Part model, mm, in its own coordinate system. A direction names the side the tool comes from. Round coordinates to 2 decimals unless told otherwise and drop trailing zeros. Write each loop counter-clockwise with the first axis right and the second up, starting at its lowest first coordinate (ties: lowest second). Pieces come first, ordered by that corner, then holes. Notation, with made-up numbers: (86.5, -10) -> (103.5, -10) arc R30 ccw to (103.5, 13) -> close; hole circle Ø5 at (-34.75, 12.5). An arc over 180 degrees is marked (long way). Use CSV: the item, a comma, the result in double quotes. Start each with the question number.
```python
from build123d import *

# Parameters (mm, degrees)
F0_W      = 114.3
F0_H      = 127
F1_DEPTH  = 304.8
F2_SIZE2  = 22.86
F2_SIZE   = 22.86
F4_D      = 63.5
F5_R      = 44.45
F5_R_2    = 31.75
F6_DEPTH  = 63.5
F8_W      = 55.88
F8_H      = 99.06
F9_DEPTH  = 147.32
F11_DEPTH = 55.88
F13_DEPTH = 302.261
F14_R     = 22.86
F15_DEPTH = 208.28


with BuildPart() as f1:
    # F0 (on Front) → F1 (new body)
    with BuildSketch(Plane.XZ):
        Rectangle(F0_W, F0_H)
    extrude(amount=-F1_DEPTH)

    # F2
    f2_edges = [f1.edges().sort_by_distance(p)[0] for p in [
        (57.15, 152.4, -63.5),
        (-57.15, 152.4, -63.5),
    ]]
    chamfer(f2_edges, length=F2_SIZE, length2=F2_SIZE2)

    # F4 (through all)
    with Locations(Plane.XZ):
        with Locations((0, -5.08)):
            Hole(F4_D / 2)

    # F5 (on face) → F6 (join)
    with BuildSketch(Plane(origin=(0, 304.8, 0), x_dir=(-1, 0, 0), z_dir=(0, 1, 0))):
        with Locations((0, -5.08)):
            Circle(F5_R)
        with Locations((0, -5.08)):
            Circle(F5_R_2, mode=Mode.SUBTRACT)
    extrude(amount=F6_DEPTH)

    # F8 (on offset) → F9 (join)
    with BuildSketch(Plane.XZ.offset(-154.94)):
        with Locations((0, -113.03)):
            Rectangle(F8_W, F8_H)
    extrude(amount=-F9_DEPTH)

    # F10 (on face) → F11 (join)
    with BuildSketch(Plane(origin=(-27.94, 0, 0), x_dir=(0, -1, 0), z_dir=(-1, 0, 0))):
        Polygon((-214.4107755243, -182.4833633625), (-203.3772818135, -168.8581333524), (-189.7520518034, -179.8916270632), (-177.4465882231, -164.6956450781), (-164.8980907601, -174.8572179642), (-154.94, -162.56), (-302.26, -162.56), (-291.6130993959, -174.939645827), (-279.7122911913, -164.7045612509), (-266.5302445016, -180.0319391764), (-253.5688132322, -168.8846840497), (-241.828860398, -182.5352724715), (-229.6067575095, -170.1778997822), align=None)
    extrude(amount=-F11_DEPTH)

    # F12 (on face) → F13 (cut, through all)
    with BuildSketch(Plane(origin=(0, 302.26, 0), x_dir=(-1, 0, 0), z_dir=(0, 1, 0))):
        Polygon((-13.8513900767, -186.9621881951), (-27.94, -162.56), (-27.94, -186.9621881951), align=None)
        Polygon((27.94, -186.9621881951), (27.94, -162.56), (13.8513900767, -186.9621881951), align=None)
    extrude(amount=-F13_DEPTH, mode=Mode.SUBTRACT)

    # F14 (on face) → F15 (cut)
    with BuildSketch(Plane.XY.offset(63.5)):
        with Locations((0, 243.84)):
            Circle(F14_R)
    extrude(amount=-F15_DEPTH, mode=Mode.SUBTRACT)


solid = f1.part
```
1. Band-saw the part on D-D (x = 38). List the corners of the cut face in (y, z).
2. Drill centre lines: line 1 along X through (y, z) = (243, 45); line 2 along Y through (x, z) = (0.5, -95); line 3 along X through (y, z) = (243.84, -117). Where is each one in solid material? Low to high. Write a range as [from, to].
3. Pull direction Y, two halves, no side cores. Call faces 1 (the flat face through (-24.8, 229.6, -168)), 2 (the flat face through (-0.391, 159.989, -168.795)), 3 (the flat face through (0, 244, -144.78)), 4 (the flat face through (-0.33, 235.8, -176.44)): released by +Y, released by -Y, zero draft, split by the parting line, or undercut.
4. Flat gauge pins, fed straight in: pin 1 (8 mm diameter, centred on x = -17, y = 196, fed in from -Z); pin 2 (4 mm diameter, centred on x = 4.5, y = 195.5, fed in from -Z); pin 3 (20.5 mm diameter, centred on x = -3, y = 124, fed in from -Z). Where does each tip first touch, or does it go through?
5. Band-saw the part on B-B (z = -106.5). List the corners of the cut face in (x, y).
6. Band-saw the part on C-C (x = 0). Give the number of separate pieces and of enclosed holes in the cut face, then the cut area to 3 significant figures.
7. Band-saw the part on A-A (z = -5.08). List the corners of the cut face in (x, y).
8. Which spindle directions (+Z, -Z, +X, -X, +Y, -Y) get a long thin tool onto all of the face, cutting with end or side? Do faces 5 (the flat face through (0, 154.94, -112)), 6 (the flat face through (-0.34, 247.781, -175.614)), 7 (the cylindrical face through (-22.838, 244.845, -85.123)). Say none if no direction does.
Answers below:
1,outline,"(0, -59.79) -> (304.8, -59.79) -> (304.8, -28.14) -> (368.3, -28.14) -> (368.3, 17.98) -> (304.8, 17.98) -> (304.8, 63.5) -> (0, 63.5) -> close"
2,line 1,"x = [-57.15, -22.84], [22.84, 57.15]"
2,line 2,"y = [154.94, 220.99], [266.69, 302.26]"
2,line 3,"x = [-27.94, -22.86], [22.86, 27.94]"
3,face 1,"zero draft"
3,face 2,"released by -Y"
3,face 3,"undercut"
3,face 4,"undercut"
4,pin 1,"stops at z = -178.07"
4,pin 2,"stops at z = -176.86"
4,pin 3,"stops at z = -63.5"
5,outline,"(-27.94, 154.94) -> (27.94, 154.94) -> (27.94, 302.26) -> (-27.94, 302.26) -> close; hole circle Ø45.72 at (0, 243.84)"
6,separate pieces,"3"
6,enclosed holes,"0"
6,area,"30,500 mm^2"
7,outline,"(-57.15, 0) -> (-31.75, 0) -> (-31.75, 368.3) -> (-44.45, 368.3) -> (-44.45, 304.8) -> (-57.15, 304.8) -> close; (31.75, 0) -> (57.15, 0) -> (57.15, 304.8) -> (44.45, 304.8) -> (44.45, 368.3) -> (31.75, 368.3) -> close"
8,face 5,"-Z, +X, -X, -Y"
8,face 6,"-Z, +X, -X"
8,face 7,"+Z"
